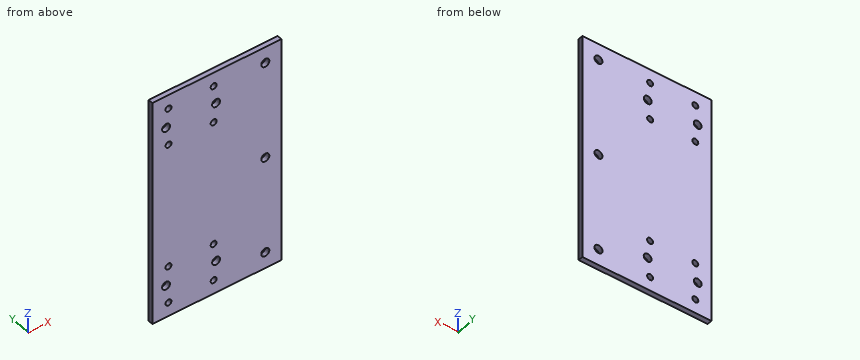
```python
from build123d import *

# Parameters (mm, degrees)
SKETCH_1_R      = 2.5
SKETCH_1_R_2    = 2.45
SKETCH_1_R_3    = 1.85
SKETCH_1_W      = 48
SKETCH_1_H      = 40
EXTRUDE_1_DEPTH = 3


with BuildPart() as part:
    # 草图1 → 凸台-拉伸1 (new body)
    # profile 1 of 5: a face of its own
    with BuildSketch(Plane(origin=(0, 0, 0), x_dir=(1, 0, 0), z_dir=(0, 1, 0))):
        with BuildLine():
            Line((8, -30), (8, -70))
            Line((8, -70), (40, -70))
            Line((40, -70), (40, 60))
            Line((40, 60), (32.5, 60))
            ThreePointArc((32.5, 60), (28.232233047, 58.232233047), (30, 62.5))
            Line((30, 62.5), (30, 70))
            Line((30, 70), (8, 70))
            Line((8, 70), (8, 30))
            Line((8, 30), (-40, 30))
            Line((-40, 30), (-40, -30))
            Line((-40, -30), (8, -30))
        make_face()
        with Locations(Location((30, -60, 0), (0, 0, 270))):
            Circle(SKETCH_1_R, mode=Mode.SUBTRACT)
        with Locations(Location((30, 0, 0), (0, 0, 270))):
            Circle(SKETCH_1_R, mode=Mode.SUBTRACT)
    # profile 2 of 5: a face of its own
    with BuildSketch(Plane(origin=(0, 0, 0), x_dir=(1, 0, 0), z_dir=(0, 1, 0))):
        with BuildLine():
            Line((32.5, 60), (40, 60))
            Line((40, 60), (40, 70))
            Line((40, 70), (30, 70))
            Line((30, 70), (30, 62.5))
            ThreePointArc((30, 62.5), (31.767766953, 61.767766953), (32.5, 60))
        make_face()
    # profile 3 of 5: a face of its own
    with BuildSketch(Plane(origin=(0, 0, 0), x_dir=(1, 0, 0), z_dir=(0, 1, 0))):
        with BuildLine():
            Line((-40, 61.45), (-40, 30))
            Line((-40, 30), (8, 30))
            Line((8, 30), (8, 70))
            Line((8, 70), (-30, 70))
            Line((-30, 70), (-30, 63.3))
            ThreePointArc((-30, 63.3), (-28.691852455, 62.758147545), (-28.15, 61.45))
            ThreePointArc((-28.15, 61.45), (-30, 59.6), (-31.85, 61.45))
            Line((-31.85, 61.45), (-40, 61.45))
        make_face()
        with Locations(Location((-31.5, 50, 0), (0, 0, 270))):
            Circle(SKETCH_1_R_2, mode=Mode.SUBTRACT)
        with Locations(Location((-30, 38.55, 0), (0, 0, 270))):
            Circle(SKETCH_1_R_3, mode=Mode.SUBTRACT)
        with Locations(Location((-2, 38.55, 0), (0, 0, 270))):
            Circle(SKETCH_1_R_3, mode=Mode.SUBTRACT)
        with Locations(Location((-0.5, 50, 0), (0, 0, 270))):
            Circle(SKETCH_1_R_2, mode=Mode.SUBTRACT)
        with Locations(Location((-2, 61.45, 0), (0, 0, 270))):
            Circle(SKETCH_1_R_3, mode=Mode.SUBTRACT)
    # profile 4 of 5: a face of its own
    with BuildSketch(Plane(origin=(0, 0, 0), x_dir=(1, 0, 0), z_dir=(0, 1, 0))):
        with BuildLine():
            Line((-40, 70), (-40, 61.45))
            Line((-40, 61.45), (-31.85, 61.45))
            ThreePointArc((-31.85, 61.45), (-31.308147545, 62.758147545), (-30, 63.3))
            Line((-30, 63.3), (-30, 70))
            Line((-30, 70), (-40, 70))
        make_face()
    # profile 5 of 5: a face of its own
    with BuildSketch(Plane(origin=(0, 0, 0), x_dir=(1, 0, 0), z_dir=(0, 1, 0))):
        with Locations((-16, -50)):
            Rectangle(SKETCH_1_W, SKETCH_1_H)
        with Locations(Location((-30, -61.45, 0), (0, 0, 270))):
            Circle(SKETCH_1_R_3, mode=Mode.SUBTRACT)
        with Locations(Location((-31.5, -50, 0), (0, 0, 270))):
            Circle(SKETCH_1_R_2, mode=Mode.SUBTRACT)
        with Locations(Location((-30, -38.55, 0), (0, 0, 270))):
            Circle(SKETCH_1_R_3, mode=Mode.SUBTRACT)
        with Locations(Location((-2, -61.45, 0), (0, 0, 270))):
            Circle(SKETCH_1_R_3, mode=Mode.SUBTRACT)
        with Locations(Location((-0.5, -50, 0), (0, 0, 270))):
            Circle(SKETCH_1_R_2, mode=Mode.SUBTRACT)
        with Locations(Location((-2, -38.55, 0), (0, 0, 270))):
            Circle(SKETCH_1_R_3, mode=Mode.SUBTRACT)
    extrude(amount=EXTRUDE_1_DEPTH)


solid = part.part
```
Input: part model. Units: mm. Frame: model coordinates. Coordinates: 2 decimals unless noted, no trailing zeros. Write each loop counter-clockwise with the first axis right and the second up, starting at its lowest first coordinate (ties: lowest second). Pieces come first, ordered by that corner, then holes. Notation, with made-up numbers: M -34,77.25 L -14,77.25 A4 cw -14,84.25 Z; hole C 27.25,0.25 d5. An arc over 180 degrees is marked long. Use one line per item in the form item = value.
Q1. First-contact query: pin 1 (5 mm diameter, centred on x = -8.5, z = -44, fed in from -Y). Flat tip, straight axial feed; report the tip coordinate or a pass-through.
Answer below:
pin_1 = 0
Q2. Section B-B (y = 1.2). Count the separate pieces of the cut face and the enclosed holes in it, plus the area to 3 significant figures.
Answer below:
separate_pieces = 1
enclosed_holes = 15
area = 11,000 mm²
Q3. Material intervals for probe 1 along X at (y, z) = (1.65, 50); probe 2 along Z at (x, y) = (28, 1.6); probe 3 along X at (y, z) = (1, -37.5), sorted ascending. Write a range as from..to.
Answer below:
probe_1 = -40..-33.95, -29.05..-2.95, 1.95..40
probe_2 = -70..-61.5, -58.5..-1.5, 1.5..58.5, 61.5..70
probe_3 = -40..-31.52, -28.48..-3.52, -0.48..40
Q4. Section C-C (z = -50). Return loops of the section in (x, y), plus the area to 3 significant figures.
Answer below:
outline = M -40,0 L -33.95,0 L -33.95,3 L -40,3 Z; M -29.05,0 L -2.95,0 L -2.95,3 L -29.05,3 Z; M 1.95,0 L 40,0 L 40,3 L 1.95,3 Z
area = 211 mm²
Q5. Section A-A (z = 38.55). Return loops of the section in (x, y).
Answer below:
outline = M -40,0 L -31.85,0 L -31.85,3 L -40,3 Z; M -28.15,0 L -3.85,0 L -3.85,3 L -28.15,3 Z; M -0.15,0 L 40,0 L 40,3 L -0.15,3 Z
